Could you check a few things on this model? Use its own coordinates, in mm. A direction names the side the tool comes from. Round coordinates to 2 decimals unless told otherwise and drop trailing zeros. Write each loop counter-clockwise with the first axis right and the second up, starting at its lowest first coordinate (ties: lowest second). Pieces come first, ordered by that corner, then holes. Notation, with made-up numbers: (87.5, 43) -> (93.5, 43) arc R25 cw to (93.5, 80) -> close; hole circle Ø3 at (23, -40). An arc over 180 degrees is marked (long way). Answer as CSV lines item,"result". Start each with the question number.
Q1. Will these pins go through, and if not, where does the flat tip stop? pin 1 Ø12 at (x, z) = (58.5, 3.5) entering from +Y; pin 2 Ø2 at (y, z) = (22, 19.5) entering from -X; pin 3 Ø5.5 at (y, z) = (-101, 11) entering from +X; pin 4 Ø6 at (y, z) = (97.93, 12.7) entering from -X.
Q2. Imagine slicing it at B-B on y = 0. Please give me the cut outline in (x, z) (3 decimals), and give its area (3 significant figures).
Q3. For faces 1 (the flat face through (12.7, -102, 13)), 2 (the flat face through (11.291, -95.189, 23.634)), 3 (the flat face through (10.842, -94.737, 1.317)), 4 (the flat face through (11.291, 94.737, 23.634)), 5 (the flat face through (12.7, 102, 13)), which set-ups out of +Z, -Z, +X, -X, +Y, -Y let a thin tool reach every point of the face, with its end or its side?
Q4. If I drill on line 1 (Y direction, x = 7.25, z = 12.7); line 2 (Y direction, x = 8.5, z = 12.7); line 3 (Y direction, x = 43, z = 11), over which ranges is the centre line in solid material (lowest first)? Write a range as [from, to].
Q5. Imagine slicing it at A-A on z = 12.7. Please give me the cut outline in (x, y) (3 decimals), and give its area (3 significant figures).
Autodesk Inventor part; units mm, degrees
ref_plane "YZ Plane" through (0, 0, 0) normal (1, 0, 0) x (0, 1, 0)
ref_plane "XZ Plane" through (0, 0, 0) normal (0, 1, 0) x (-1, 0, 0)
ref_plane "XY Plane" through (0, 0, 0) normal (0, 0, 1) x (1, 0, 0)
sketch "Sketch1" plane through (0, 0, 0) normal (0, 0, 1) x (1, 0, 0)
  circle A0 centre (0, 0) radius 56.515
  line L0 (12.7, -114.3) -> (-12.7, -114.3)
  line L1 (-12.7, 114.3) -> (12.7, 114.3)
  line L2 (12.7, 114.3) -> (-12.7, -114.3) construction
  line L3 (12.7, -114.3) -> (-12.7, 114.3) construction
  line L4 (12.7, -81.5672) -> (12.7, -114.3)
  line L5 (-12.7, -114.3) -> (-12.7, -81.5672)
  line L6 (12.7, 114.3) -> (12.7, 81.5672)
  arc A1 (12.7, -81.5672) -> (12.7, 81.5672) centre (0, 0) ccw
  arc A2 (-12.7, 81.5672) -> (-12.7, -81.5672) centre (0, 0) ccw
  line L7 (-12.7, 81.5672) -> (-12.7, 114.3)
  line L8 (0, 114.3) -> (0, -114.3)
  line L9 (-0.7937, -114.3) -> (0.7937, -114.3)
  line L10 (0.7937, -114.3) -> (0.7937, 114.3)
  line L11 (0.7937, 114.3) -> (-0.7937, 114.3)
  line L12 (-0.7937, 114.3) -> (-0.7937, -114.3)
  line L13 (-0.7937, -114.3) -> (0.7937, 114.3) construction
  line L14 (0.7937, -114.3) -> (-0.7937, 114.3) construction
  dimension "d0" = 113.03
  dimension "d1" = 228.6
  dimension "d2" = 25.4
  dimension "d3" = 82.55
  dimension "d4" = 82.55
  dimension "d5" = 32.7328
  dimension "d6" = 32.7328
  dimension "d7" = 1.5875
extrude "Extrusion1" add sketch "Sketch1" along normal blind 25.4 contours A0 L10 | A0 L10 L1 L6 A1 L4 L0 | L10 A0 L8 | A0 L8 L1 L10 | L10 L0 L8 A0
sketch "Sketch2" plane through (0, 0, 25.4) normal (0, 0, 1) x (1, 0, 0)
  arc A0 (12.7, -81.5672) -> (12.7, 81.5672) centre (0, 0) ccw
  circle A1 centre (0, 0) radius 56.515
  dimension "d10" = 113.03
extrude "Extrusion2" cut sketch "Sketch2" against normal blind 25.4
sketch "Sketch3" plane through (12.7, 81.5672, 0) normal (1, 0, 0) x (0, 0, -1)
  line L0 (-25.4, 32.7328) -> (0, 0) construction
  line L1 (0, -138.0822) -> (0, -195.8672)
  line L2 (-25.4, -163.1345) -> (0, -195.8672) construction
  point P0 (0, -81.5672)
  point P1 (-12.7, -179.5008)
  point P2 (-12.7, 16.3664)
hole "Hole1" at (12.7, -97.9336, 12.7) at (12.7, 97.9336, 12.7) direction (-1, 0, 0) diameter 6.858 depth 15.6718 tip angle 118
chamfer "Chamfer1" distance 3.175 angle 45 14 edges at (56.515, 0, 25.4) (56.515, 0, 0) (82.55, 0, 0) (82.55, 0, 25.4) (12.7, 97.9336, 25.4) (12.7, 114.3, 12.7) (12.7, 97.9336, 0) (12.7, -97.9336, 0) (12.7, -97.9336, 25.4) (12.7, -114.3, 12.7) (6.35, -114.3, 25.4) (6.35, -114.3, 0) (6.35, 114.3, 25.4) (6.35, 114.3, 0)
fillet "Fillet1" radius 6.35 2 edges at (12.7, -81.5672, 12.7) (12.7, 81.5672, 12.7)
equation "\"d4\" = d3"
equation "\"d6\" = d5"
properties part number "2122_Copper Tube Clamp Top_V1" material "ABS Plastic"
Checks:
1,pin 1,"y = 63.7"
1,pin 2,"x = 51.62"
1,pin 3,"x = 12.7"
1,pin 4,"through"
2,outline,"(56.515, 3.175) -> (59.69, 0) -> (79.375, 0) -> (82.55, 3.175) -> (82.55, 22.225) -> (79.375, 25.4) -> (59.69, 25.4) -> (56.515, 22.225) -> close"
2,area,"641 mm^2"
3,face 1,"+Z, -Z, +X, -Y"
3,face 2,"+Z, +X, -Y"
3,face 3,"-Z, +X, -Y"
3,face 4,"+Z, +X, +Y"
3,face 5,"+Z, -Z, +X, +Y"
4,line 1,"[-114.3, -101.36], [-94.5, -56.05], [56.05, 94.5], [101.36, 114.3]"
4,line 2,"[-114.3, -101.36], [-94.5, -55.87], [55.87, 94.5], [101.36, 114.3]"
4,line 3,"[-70.47, -36.67], [36.67, 70.47]"
5,outline,"(0, -114.3) -> (9.525, -114.3) -> (12.7, -111.125) -> (12.7, -101.363) -> (0, -101.363) -> close; (0, -94.505) -> (12.7, -94.505) -> (12.7, -86.835) arc R6.35 cw to (17.689, -80.632) arc R82.55 ccw to (17.689, 80.632) arc R6.35 cw to (12.7, 86.835) -> (12.7, 94.505) -> (0, 94.505) -> (0, 56.515) arc R56.515 cw to (0, -56.515) -> close; (0, 101.363) -> (12.7, 101.363) -> (12.7, 111.125) -> (9.525, 114.3) -> (0, 114.3) -> close"
5,area,"6,330 mm^2"
